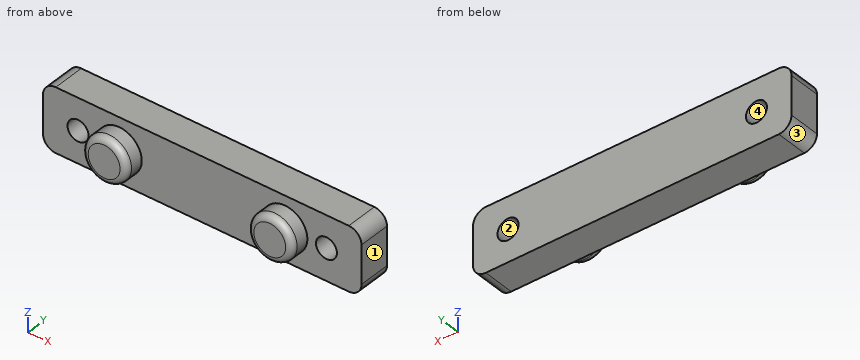
Autodesk Inventor part; units mm, degrees
ref_plane "YZ Plane" through (0, 0, 0) normal (1, 0, 0) x (0, 1, 0)
ref_plane "XZ Plane" through (0, 0, 0) normal (0, 1, 0) x (-1, 0, 0)
ref_plane "XY Plane" through (0, 0, 0) normal (0, 0, 1) x (1, 0, 0)
sketch "Эскиз1" plane through (0, 0, 0) normal (0, 1, 0) x (-1, 0, 0)
  circle A0 centre (0, 0) radius 3.5
  circle A1 centre (-26, 0) radius 3.5
  line L0 (-3.5, 0) -> (-22.5, 0) construction
  line L1 (0, 0) -> (-26, 0) construction
  circle A2 centre (-32.5, 0) radius 1.65
  circle A3 centre (6.5, 0) radius 1.65
  line L2 (10, -5) -> (-36, -5)
  line L3 (-38, -3) -> (-38, 3)
  line L4 (-36, 5) -> (10, 5)
  line L5 (12, 3) -> (12, -3)
  arc A4 (10, -5) -> (12, -3) centre (10, -3) ccw
  arc A5 (12, 3) -> (10, 5) centre (10, 3) ccw
  arc A6 (-38, -3) -> (-36, -5) centre (-36, -3) ccw
  arc A7 (-36, 5) -> (-38, 3) centre (-36, 3) ccw
  circle A8 centre (-32.5, 0) radius 3.65
  circle A9 centre (6.5, 0) radius 3.65
  point P0 (3.5, 0)
  point P1 (4.85, 0)
  point P2 (-29.5, 0)
  point P3 (-30.85, 0)
  point P4 (-29.5, 0)
  point P5 (-30.85, 0)
  point P6 (-29.5, 0)
  point P7 (-30.85, 0)
  point P8 (-29.5, 0)
  point P9 (-30.85, 0)
  dimension "d4" = 3.3
  dimension "d5" = 3.3
  dimension "d0" = 7
  dimension "d1" = 7
  dimension "d3" = 19
  dimension "d8" = 3
  dimension "d9" = 3
  dimension "d10" = 12
  dimension "d11" = 12
  dimension "d12" = 5
  dimension "d13" = 10
  dimension "d14" = 2
  dimension "d15" = 2
  dimension "d16" = 2
extrude "Выдавливание1" add sketch "Эскиз1" along normal blind 5 contours A0 A9 | A0 A9 | A9 A0 | A1 A8 | A8 A1 | A1 A8 | L2 A6 L3 A7 L4 A5 L5 A4
extrude "Выдавливание2" add sketch "Эскиз1" against normal blind 3 contours A0 A9 | A9 A0 | A1 A8 | A8 A1 picked at (3.0809, 0.424) picked at (-1.3483, -0.2837) picked at (-24.6517, 0.2837) picked at (-29.2672, -0.4241)
fillet "Сопряжение1" radius 1 2 edges at (3.5, -3, 0) (29.5, -3, 0)
properties part number "Conductor_Volume_Encoder"
Read the model definition and answer for the solid it produces. Units are mm, in the model's axes. Face numbers are marked on the shaded views. Coordinates: 2 decimals unless noted, no trailing zeros. Order: outer loops, then holes, each group sorted by start corner. A loop starts at its lowest first (then second) coordinate and runs counter-clockwise, first axis right, second up. Notation, with made-up numbers: (-25, 50) - (3, 50) arc R30 ccw to (3, 89) - close; hole circle Ø5 at (47, 78.5). An arc over 180 degrees is marked (long way). Answer as a JSON object with one key per item and string values. Group by question number.
Item 1: Section D-D (x = 26) is taken. Give the vertices of the cut face in (y, z), plus the area to 3 significant figures.
Item 2: Section C-C (z = 0) is taken. Give the vertices of the cut face in (x, y).
Item 3: Consider probe 1 along Z at (x, y) = (32.5, 1.45); probe 2 along X at (y, z) = (4, 0.5); probe 3 along Y at (x, z) = (20.5, -1.75). Determine where each line is inside the solid, lowest interval first. Write a range as from..to.
Item 4: Section A-A (x = -6.5) is taken. Give the vertices of the cut face in (y, z), plus the area to 3 significant figures.
Item 5: The mould has two halves that part along Z. Classify the marked faces 1, 2, 3 and 4: +Z half, -Z half, draft (parallel to the pull), parting line (faces both ways), or undercut.
Item 6: A flat-ended cylindrical pin translates along its axis: P1, Ø4.5, axis at x = 32.5, z = 0, coming from the -Y side. Find the tip coordinate at first contact, or state that the pin passes through.
Item 7: Section B-B (y = 3) is taken. Give the vertices of the cut face in (x, z), plus the area to 3 significant figures.
Results are:
{
 "1": {"outline": "(-3, -2.5) arc R1 ccw to (-2, -3.5) - (0, -3.5) - (0, -5) - (5, -5) - (5, 5) - (0, 5) - (0, 3.5) - (-2, 3.5) arc R1 ccw to (-3, 2.5) - close", "area": "70.6 mm^2"},
 "2": {"outline": "(-12, 0) - (-8.15, 0) - (-8.15, 5) - (-12, 5) - close; (-4.85, 0) - (-3.5, 0) - (-3.5, -2) arc R1 ccw to (-2.5, -3) - (2.5, -3) arc R1 ccw to (3.5, -2) - (3.5, 0) - (22.5, 0) - (22.5, -2) arc R1 ccw to (23.5, -3) - (28.5, -3) arc R1 ccw to (29.5, -2) - (29.5, 0) - (30.85, 0) - (30.85, 5) - (-4.85, 5) - close; (34.15, 0) - (38, 0) - (38, 5) - (34.15, 5) - close"},
 "3": {"probe 1": "z = -5..-1.65, 1.65..5", "probe 2": "x = -12..-8.07, -4.93..30.93, 34.07..38", "probe 3": "y = 0..5"},
 "4": {"outline": "(0, -5) - (5, -5) - (5, -1.65) - (0, -1.65) - close; (0, 1.65) - (5, 1.65) - (5, 5) - (0, 5) - close", "area": "33.5 mm^2"},
 "5": {"face 1": "draft", "face 2": "undercut", "face 3": "-Z half", "face 4": "undercut"},
 "6": {"P1": "stops at y = 0"},
 "7": {"outline": "(-12, -3) arc R2 ccw to (-10, -5) - (36, -5) arc R2 ccw to (38, -3) - (38, 3) arc R2 ccw to (36, 5) - (-10, 5) arc R2 ccw to (-12, 3) - close; hole circle Ø3.3 at (-6.5, 0); hole circle Ø3.3 at (32.5, 0)", "area": "479 mm^2"}
}
